Geometry check sheet. Reference: drawing and pictorial views, mm from the part's lowest x, y, z. Coordinates: 2 decimals unless noted, no trailing zeros. Loops run counter-clockwise (first coordinate to the right, second up) from the corner with the lowest first, then second, coordinate; pieces in that order, holes last. Notation, with made-up numbers: (0, 43) - (44, 43) arc R21 ccw to (44, 69) - close; hole circle Ø3 at (44, 46). An arc over 180 degrees is marked (long way). One line per item, written item: value.
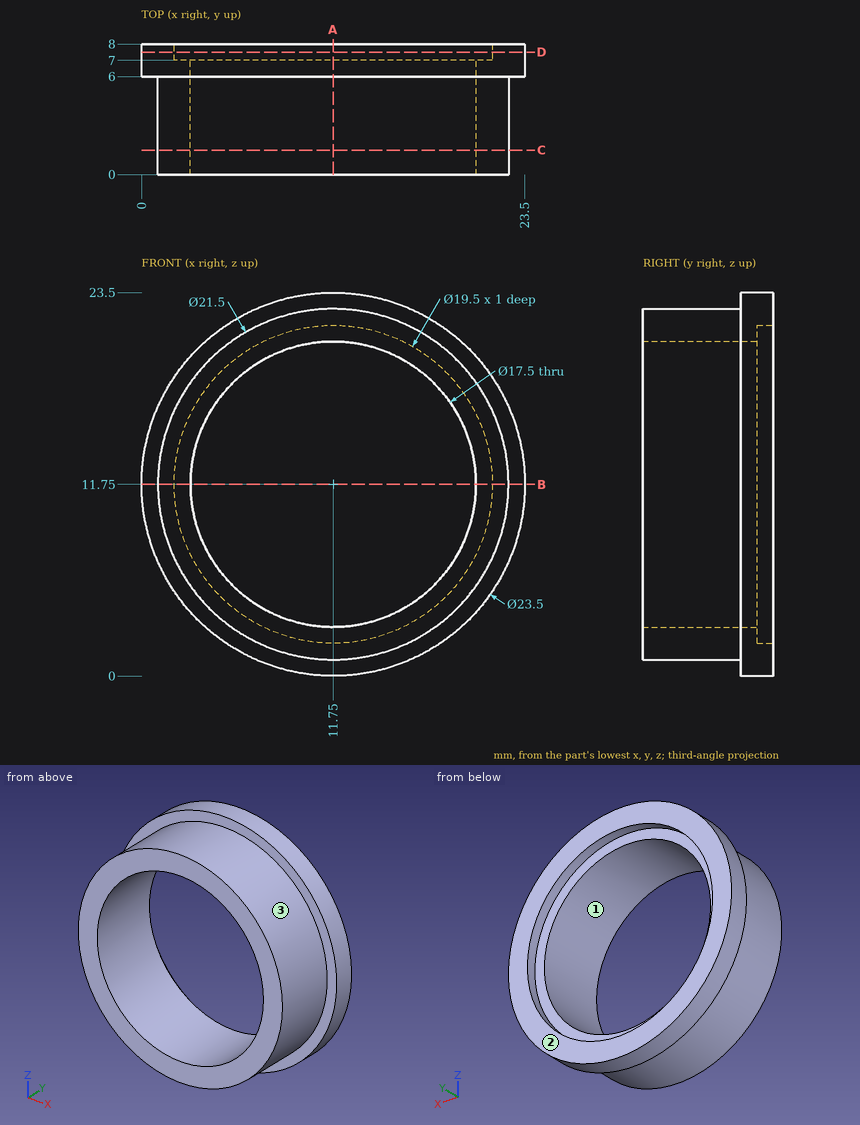
(1) Material ranges on probe 1 along Z at (x, y) = (11.75, 7.3); probe 2 along Y at (x, z) = (10, 2.5); probe 3 along Z at (x, y) = (6, 1.25), recorded low to high. Write a range as from..to.
Reply:
probe 1: 0..2, 21.5..23.5
probe 2: 0..7
probe 3: 2.67..5.15, 18.35..20.83
(2) Cross-section at A-A on x = 11.75. Record the cut outline in (y, z), and give its area (3 significant figures).
Reply:
outline: (0, 1) - (6, 1) - (6, 0) - (8, 0) - (8, 2) - (7, 2) - (7, 3) - (0, 3) - close; (0, 20.5) - (7, 20.5) - (7, 21.5) - (8, 21.5) - (8, 23.5) - (6, 23.5) - (6, 22.5) - (0, 22.5) - close
area: 34.0 mm2
(3) Go/stop test with flat-tipped pins: pin 1 Ø2 at (y, z) = (2.5, 19) entering from +X; pin 2 Ø10 at (x, z) = (8, 13) entering from +Y. Record where each tip stops, or that it passes through.
Reply:
pin 1: x = 20.5
pin 2: y = 7
(4) Cross-section at B-B on z = 11.75. Record the cut outline in (x, y).
Reply:
outline: (0, 6) - (1, 6) - (1, 0) - (3, 0) - (3, 7) - (2, 7) - (2, 8) - (0, 8) - close; (20.5, 0) - (22.5, 0) - (22.5, 6) - (23.5, 6) - (23.5, 8) - (21.5, 8) - (21.5, 7) - (20.5, 7) - close
(5) Release check for a two-part mould opening along Z. For the marked faces 1, 2 and 3 record: pulls with the +Z half, pulls with the -Z half, needs draft (parallel to the pull), parting line crosses it, or undercut.
Reply:
face 1: undercut
face 2: needs draft
face 3: parting line crosses it
(6) Cross-section at D-D on y = 7.5. Record the cut outline in (x, z).
Reply:
outline: circle Ø23.5 at (11.75, 11.75); hole circle Ø19.5 at (11.75, 11.75)
(7) Cross-section at C-C on y = 1.5. Record the cut outline in (x, z), and give its area (3 significant figures).
Reply:
outline: circle Ø21.5 at (11.75, 11.75); hole circle Ø17.5 at (11.75, 11.75)
area: 123 mm2
